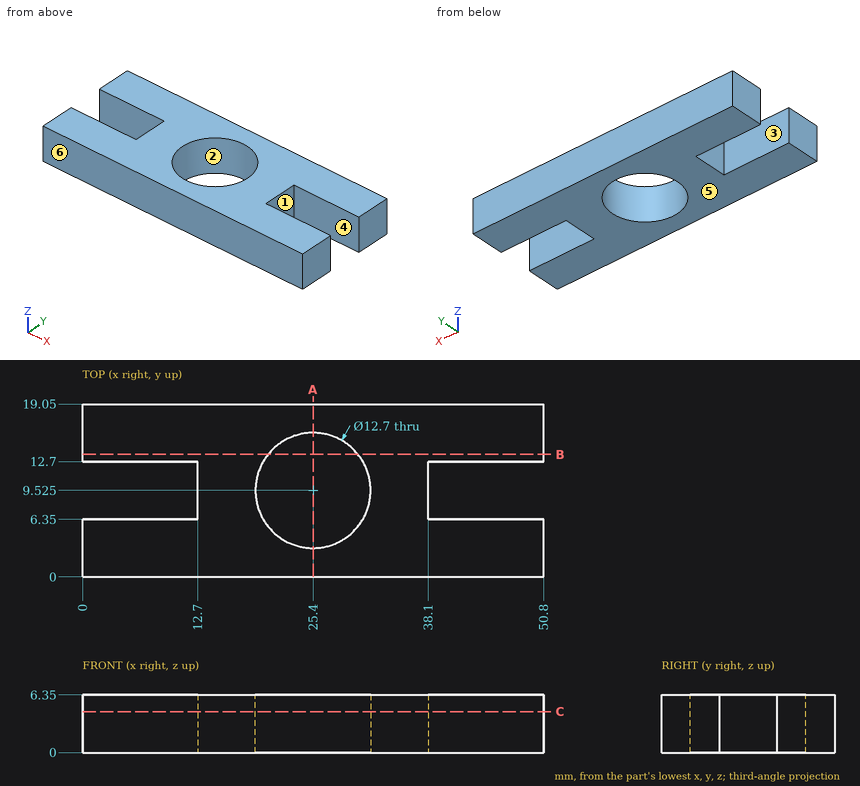
Can you work these out from the drawing? Everything is in mm from the part's minimum corner. A direction names the side the tool comes from. Round coordinates to 2 decimals unless told otherwise and drop trailing zeros. Loops run counter-clockwise (first coordinate to the right, second up) from the corner with the lowest first, then second, coordinate; pieces in that order, holes last. Notation, with made-up numbers: (22, 39.5) - (42, 39.5) arc R10 cw to (42, 43.5) - close; hole circle Ø5 at (73.5, 75). An arc over 180 degrees is marked (long way). Answer in a Markdown table with one row per item. Add a question column.
Q1. I want a section at B-B on y = 13.5. List the corners of the cut face in (x, z) for me.
Q2. I need wall thicknesses on L1, parallel to Y at x = 25.4, z = 3.75 (3 decimals); L2, parallel to Y at x = 41.5, z = 5; L3, parallel to X at y = 6, z = 4.5. Which ranges of each line are inside material? Lowest first, please.
Q3. We'd pull the mould along Y, two halves only. Please class the marked faces 4, 5 and 6: pulls with the +Y half, pulls with the -Y half, needs draft (parallel to the pull), parting line crosses it, or undercut.
Q4. Which directions (+Z, -Z, +X, -X, +Y, -Y) give clear straight access to the entire face, cutting with the end or side of a thin tool? Please do the marked faces 1, 2 and 3.
Q5. I want a section at C-C on z = 4.5. List the corners of the cut face in (x, y) for me (3 decimals).
Q6. For pin 1 Ø1.9 at (y, z) = (11, 3.5) entering from -X, with a flat end and sliding along its axis, tell me the tip position at first contact or that it passes through.
Q7. I want a section at A-A on x = 25.4. List the corners of the cut face in (y, z) for me (3 decimals).
A:
| question | item | result |
|---|---|---|
| 1 | outline | (0, 0) - (20.45, 0) - (20.45, 6.35) - (0, 6.35) - close; (30.35, 0) - (50.8, 0) - (50.8, 6.35) - (30.35, 6.35) - close |
| 2 | L1 | 0 to 3.175, 15.875 to 19.05 |
| 2 | L2 | 0 to 6.35, 12.7 to 19.05 |
| 2 | L3 | 0 to 20.12, 30.68 to 50.8 |
| 3 | face 4 | undercut |
| 3 | face 5 | needs draft |
| 3 | face 6 | pulls with the -Y half |
| 4 | face 1 | +Z, -Z, +X |
| 4 | face 2 | +Z, -Z |
| 4 | face 3 | +Z, -Z, -X |
| 5 | outline | (0, 0) - (50.8, 0) - (50.8, 6.35) - (38.1, 6.35) - (38.1, 12.7) - (50.8, 12.7) - (50.8, 19.05) - (0, 19.05) - (0, 12.7) - (12.7, 12.7) - (12.7, 6.35) - (0, 6.35) - close; hole circle Ø12.7 at (25.4, 9.525) |
| 6 | pin 1 | x = 12.7 |
| 7 | outline | (0, 0) - (3.175, 0) - (3.175, 6.35) - (0, 6.35) - close; (15.875, 0) - (19.05, 0) - (19.05, 6.35) - (15.875, 6.35) - close |
